Could you check a few things on this drawing? It's one solid part, dimensions in mm from its lowest x, y, z. A direction names the side the tool comes from. Round coordinates to 2 decimals unless told otherwise and drop trailing zeros. Order: outer loops, then holes, each group sorted by start corner. A loop starts at its lowest first (then second) coordinate and runs counter-clockwise, first axis right, second up. Notation, with made-up numbers: (13.25, 84.5) -> (65.25, 84.5) arc R33 ccw to (65.25, 122.5) -> close; hole circle Ø1 at (86, 71.5). An arc over 180 degrees is marked (long way). Use a Markdown table: item, result. Add a question column.
(1) I want a section at C-C, the plane z = 10. Please give me the cut outline in (x, y) (1 decimal).
(2) I want a section at B-B, the plane x = 15.5. Please give me the cut outline in (y, z) (1 decimal).
(3) I'm going to push flat-ended pins straight in: P1, Ø8, axis at x = 24, z = 12, coming from the -Y side; P2, Ø5, axis at y = 8, z = 12.5, coming from the -X side; P3, Ø3, axis at y = 17, z = 3.5, coming from the -X side; P4, Ø5, axis at x = 15.5, z = 10, coming from the +Y side. Where does each tip first touch, or does it pass through?
(4) If I drill on probe 1 along X at (y, z) = (1.5, 2); probe 2 along Z at (x, y) = (17, 15.75); probe 3 along Z at (x, y) = (14.5, 13), over which ranges is the centre line in solid material (lowest first)?
(5) I want a section at A-A, the plane y = 2.75. Please give me the cut outline in (x, z).
(6) On a 3-axis mill with a long thin cutter (end or side, diameter ignored), from which of +Z, -Z, +X, -X, +Y, -Y can I reach the whole of each face in a straight line? I mean the marked faces 1, 2 and 3. Say none if no direction works.
(7) I want a section at D-D, the plane z = 2.5. Please give me the cut outline in (x, y).
(8) Thinking about a two-plate mould opening in Z: for the marked faces 4, 5 and 6, which applies, pulls with the +Z half, pulls with the -Z half, needs draft (parallel to the pull), parting line crosses it, or undercut?
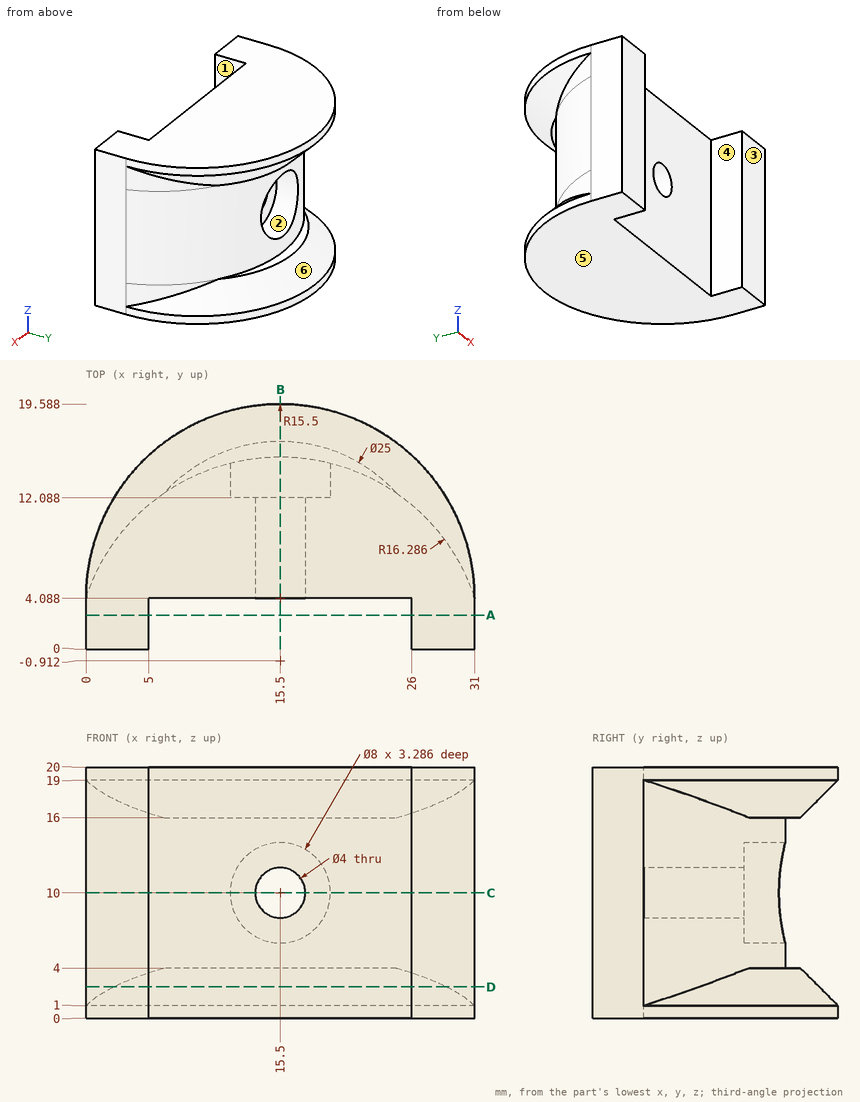
Taken from the geometry:
| question | item | result |
|---|---|---|
| 1 | outline | (0, 0) -> (5, 0) -> (5, 4.1) -> (13.5, 4.1) -> (13.5, 12.1) -> (11.5, 12.1) -> (11.5, 14.9) arc R16.3 ccw to (0, 4.1) -> close; (17.5, 4.1) -> (26, 4.1) -> (26, 0) -> (31, 0) -> (31, 4.1) arc R16.3 ccw to (19.5, 14.9) -> (19.5, 12.1) -> (17.5, 12.1) -> close |
| 2 | outline | (4.1, 0) -> (19.6, 0) -> (19.6, 1) -> (16.6, 4) -> (15.4, 4) -> (15.4, 6) -> (12.1, 6) -> (12.1, 8) -> (4.1, 8) -> close; (4.1, 12) -> (12.1, 12) -> (12.1, 14) -> (15.4, 14) -> (15.4, 16) -> (16.6, 16) -> (19.6, 19) -> (19.6, 20) -> (4.1, 20) -> close |
| 3 | P1 | stops at y = 0 |
| 3 | P2 | stops at x = 0.53 |
| 3 | P3 | stops at x = 7.92 |
| 3 | P4 | stops at y = 12.09 |
| 4 | probe 1 | x = 0 to 5, 26 to 31 |
| 4 | probe 2 | z = 0 to 4, 16 to 20 |
| 4 | probe 3 | z = 0 to 6.13, 13.87 to 20 |
| 5 | outline | (0, 0) -> (5, 0) -> (5, 20) -> (0, 20) -> close; (26, 0) -> (31, 0) -> (31, 20) -> (26, 20) -> close |
| 6 | face 1 | +Z, -Z, -Y |
| 6 | face 2 | +Y |
| 6 | face 3 | +Z, -Z, +X, -X, -Y |
| 7 | outline | (0, 0) -> (5, 0) -> (5, 4.09) -> (26, 4.09) -> (26, 0) -> (31, 0) -> (31, 4.09) arc R16.29 ccw to (28.78, 8.51) arc R14 ccw to (2.22, 8.51) arc R16.29 ccw to (0, 4.09) -> close |
| 8 | face 4 | needs draft |
| 8 | face 5 | pulls with the -Z half |
| 8 | face 6 | undercut |
